Geometry check sheet. Reference: the model listing, model coordinates, mm. A direction names the side the tool comes from. Round coordinates to 2 decimals unless told otherwise and drop trailing zeros. Order: outer loops, then holes, each group sorted by start corner. A loop starts at its lowest first (then second) coordinate and runs counter-clockwise, first axis right, second up. Notation, with made-up numbers: (-2.5, 77) - (1.5, 77) arc R10 ccw to (1.5, 93) - close; hole circle Ø4 at (37.5, 48). An arc over 180 degrees is marked (long way). Answer as CSV lines item,"result". Start each with the question number.
```python
from build123d import *

# Parameters (mm, degrees)
F0_R     = 20.32
F1_DEPTH = 50.8
F7_R     = 3.0729490934
F8_DEPTH = 78.74


with BuildPart() as f1:
    # F0 (on Top) → F1 (new body, symmetric)
    with BuildSketch(Plane.XY):
        Circle(F0_R)
    extrude(amount=F1_DEPTH, both=True)

    # F2 (on Front) → F3 (revolve)
    with BuildSketch(Plane.XZ):
        with BuildLine():
            Line((0, 50.9317442775), (20.189454779, 50.5773611367))
            ThreePointArc((20.189454779, 50.5773611367), (14.4030478755, 65.0841957818), (0, 71.1243090399))
            Line((0, 71.1243090399), (0, 50.9317442775))
        make_face()
    revolve(axis=Axis((0, 0, 61.0280266587), (0, 0, -1)))

    # F5 (on Right) → F6 (revolve)
    with BuildSketch(Plane.YZ):
        Polygon((0, 62.3119361699), (1.6591945896, 62.3119361699), (7.0054852404, 62.3119361699), (4.2401598766, 78.903876245), (0, 78.903876245), align=None)
    revolve(axis=Axis((0, 0, 70.6079062074), (0, 0, -1)))

    # F7 (on Right) → F8 (join)
    with BuildSketch(Plane.YZ):
        with Locations((2.5758331176, 74.3131265044)):
            Circle(F7_R)
    extrude(amount=F8_DEPTH)

    # F9 (on Front) → F10 (revolve)
    with BuildSketch(Plane.XZ):
        with BuildLine():
            add(Edge.make_bspline(
                [(77.1916285157, 77.2717222571), (80.5414482084, 77.6263895759), (88.7637679854, 78.496940345), (90.2856769773, 65.3756755472), (91.1875516176, 57.6000884175)],
                knots=[0, 0, 0, 0, 0.4074056694, 1, 1, 1, 1], degree=3))
            Line((77.1916285157, 77.2717222571), (79.1982337832, 74.6180936694))
            add(Edge.make_bspline(
                [(79.1982337832, 74.6180936694), (80.9350673917, 74.6645930701), (85.9177561117, 74.7979921694), (84.5073837742, 64.3036691827), (83.588629961, 57.4673898518)],
                knots=[0, 0, 0, 0, 0.3485735726, 1, 1, 1, 1], degree=3))
            Line((83.588629961, 57.4673898518), (91.1875516176, 57.6000884175))
        make_face()
        with BuildLine():
            Line((79.1982337832, 74.6180936694), (77.1916285157, 77.2717222571))
            Line((77.1916285157, 77.2717222571), (83.588629961, 57.4673898518))
            add(Edge.make_bspline(
                [(79.1982337832, 74.6180936694), (80.9350673917, 74.6645930701), (85.9177561117, 74.7979921694), (84.5073837742, 64.3036691827), (83.588629961, 57.4673898518)],
                knots=[0, 0, 0, 0, 0.3485735726, 1, 1, 1, 1], degree=3))
        make_face()
    revolve(axis=Axis((80.3901292384, 0, 67.3695560545), (0.3073729937, 0, -0.9515891144)))

    # F11 (on Front) → F12 (revolve)
    with BuildSketch(Plane.XZ):
        Polygon((91.4701148868, 57.5232356787), (83.6011469364, 57.0121742785), (83.9662040441, 54.9480340358), (90.231738364, 56.0561359902), (109.0413108468, 2.9503183905), (110.7993200421, 2.9503183905), align=None)
    revolve(axis=Axis((88.3817486465, 0, 29.9812463345), (0.1741540854, 0, -0.9847184138)))


solid = f1.part
```
1. Thickness scan on probe 1 along X at (y, z) = (-7.5, 37); probe 2 along X at (y, z) = (-6, 42.5); probe 3 along X at (y, z) = (-2, 64). Record the ranges inside material, lowest first.
2. Go/stop test with flat-tipped pins: pin 1 Ø10 at (x, y) = (79.5, 9.5) entering from +Z; pin 2 Ø12 at (x, y) = (10, 9) entering from +Z; pin 3 Ø4 at (y, z) = (-4, 43.5) entering from +X; pin 4 Ø10 at (x, y) = (71, 15) entering from -Z. Record where each tip stops, or that it passes through.
3. Section check A-A on z = -43. Record the boundary of the cut face in (x, y), plus the area to 3 significant figures.
4. Section check C-C on z = 32. Count the separate pieces of the cut face and the enclosed holes in it, plus the area to 3 significant figures.
5. Draft check along Y on faces 1 (the face through (0, 0, -50.8)), 2 (the face through (100.06, 4.8, 30.45)), 3 (the face through (85.662, -0.622, 57.476)). Enter one of: released by +Y, released by -Y, zero draft, split by the parting line, or undercut.
6. Access from +Z, -Z, +X, -X, +Y, -Y to the whole of each face (thin tool, end or side, straight path). Record for faces 4 (the face through (84.496, -0.089, 55.042)), 5 (the face through (0, 0, 78.904)), 6 (the face through (85.635, -0.637, 57.133)).
7. Section check B-B on x = 28. Record the boundary of the cut face in (y, z).
Numbers:
1,probe 1,"x = -18.89 to 18.89, 79.17 to 81.65, 93.19 to 95.77"
1,probe 2,"x = -19.41 to 19.41, 78.15 to 80.34, 92.5 to 94.8"
1,probe 3,"x = -15.26 to 15.26, 72.07 to 90.14"
2,pin 1,"stops at z = 76.66"
2,pin 2,"stops at z = 77.36"
2,pin 3,"stops at x = 96.61"
2,pin 4,"passes through"
3,outline,"circle Ø40.64 at (0, 0)"
3,area,"1,300 mm2"
4,separate pieces,"2"
4,enclosed holes,"1"
4,area,"1,420 mm2"
5,face 1,"zero draft"
5,face 2,"split by the parting line"
5,face 3,"undercut"
6,face 4,"-Z"
6,face 5,"+Z, +X, -X, +Y, -Y"
6,face 6,"none"
7,outline,"circle Ø6.15 at (2.58, 74.31)"
